Verification items for the finished model (mm, model axes). Face numbers are marked on the shaded views. A direction names the side the tool comes from. Round coordinates to 2 decimals unless told otherwise and drop trailing zeros. Write each loop counter-clockwise with the first axis right and the second up, starting at its lowest first coordinate (ties: lowest second). Pieces come first, ordered by that corner, then holes. Notation, with made-up numbers: M 83.25,34 L 127.25,34 A20 cw 127.25,48 Z; hole C 67.5,59 d7. An arc over 180 degrees is marked long. One line per question, with ' | ' between items. Start each with the question number.
Q1. Tool access check on the marked faces 4 and 5. Record the directions out of +Z, -Z, +X, -X, +Y, -Y that give a thin tool (end or side, any length) a straight path to the whole face; none if there is none.
Q2. Cross-section at C-C (x = -15). Record the boundary of the cut face in (y, z), then the cut area to 3 significant figures.
Q3. Cross-section at A-A (y = -2.75). Record the boundary of the cut face in (x, z).
Q4. Thickness scan on line 1 along X through (y, z) = (-9.5, -56.5); line 2 along Z through (x, y) = (17, -9.5); line 3 along X through (y, z) = (-13.25, -12.5). Record the ranges inside material, lowest first. Write a range as from..to.
Q5. Release check for a two-part mould opening along X. For the marked faces 1, 2 and 3 record: released by +X, released by -X, zero draft, split by the parting line, or undercut.
Q6. Gauge pin test, flat ends, axial feed: pin 1 (4 mm diameter, centred on x = 1.5, z = -57.5, fed in from -Y); pin 2 (2 mm diameter, centred on x = -6, y = -14.5, fed in from -Z). Record the tip position at first contact, or that the pin passes through.
Q7. Cross-section at D-D (z = -23.5). Record the boundary of the cut face in (x, y).
from build123d import *
from OCP.BRepFilletAPI import BRepFilletAPI_MakeChamfer

# Parameters (mm, degrees)
SKETCH1_W           = 35.4
SKETCH1_H           = 99.4
SKETCH1_W_2         = 33
SKETCH1_H_2         = 97
BOSS_EXTRUDE1_DEPTH = 2.4
SKETCH2_W           = 39.4
SKETCH2_H           = 103.4
SKETCH2_W_2         = 35.4
SKETCH2_H_2         = 99.4
BOSS_EXTRUDE3_DEPTH = 15.4
SKETCH3_W           = 39.4
SKETCH3_H           = 103.4
BOSS_EXTRUDE4_DEPTH = 2
BOSS_EXTRUDE5_DEPTH = 21.4
SKETCH5_R           = 5
CUT_EXTRUDE1_DEPTH  = 2.4
SKETCH6_W           = 4
SKETCH6_H           = 105.4
BOSS_EXTRUDE6_DEPTH = 1.6
CHAMFER1_SIZE       = 0.4
CHAMFER1_SIZE_2     = 2


with BuildPart() as part:
    # Sketch1 → Boss-Extrude1 (new body)
    with BuildSketch(Plane(origin=(0, 0, 0), x_dir=(1, 0, 0), z_dir=(0, 1, 0))):
        with Locations((0, 49.5)):
            Rectangle(SKETCH1_W, SKETCH1_H)
        with Locations((0, 49.5)):
            Rectangle(SKETCH1_W_2, SKETCH1_H_2, mode=Mode.SUBTRACT)
    extrude(amount=BOSS_EXTRUDE1_DEPTH)

    # Sketch2 → Boss-Extrude3 (add)
    with BuildSketch(Plane(origin=(0, 2.4, 0), x_dir=(1, 0, 0), z_dir=(0, 1, 0))):
        with Locations((0, 49.5)):
            Rectangle(SKETCH2_W, SKETCH2_H)
        with Locations((0, 49.5)):
            Rectangle(SKETCH2_W_2, SKETCH2_H_2, mode=Mode.SUBTRACT)
    extrude(amount=-BOSS_EXTRUDE3_DEPTH)

    # Sketch3 → Boss-Extrude4 (add)
    with BuildSketch(Plane(origin=(0, 2.4, 0), x_dir=(1, 0, 0), z_dir=(0, 1, 0))):
        with Locations((0, 49.5)):
            Rectangle(SKETCH3_W, SKETCH3_H)
    extrude(amount=BOSS_EXTRUDE4_DEPTH)

    # Sketch4 → Boss-Extrude5 (add)
    with BuildSketch(Plane(origin=(0, 4.4, 0), x_dir=(1, 0, 0), z_dir=(0, 1, 0))):
        Polygon((21.7, 101.2), (21.7, -4.2), (-21.7, -4.2), (-21.7, 101.2), (-19.7, 101.2), (-19.7, -2.2), (19.7, -2.2), (19.7, 101.2), align=None)
    extrude(amount=-BOSS_EXTRUDE5_DEPTH)

    # Sketch5 → Cut-Extrude1 (cut)
    with BuildSketch(Plane.XZ.offset(13)):
        with Locations((-15.2, -23.2)):
            Circle(SKETCH5_R)
        with Locations((15.2, -23.2)):
            Circle(SKETCH5_R)
        with Locations((15.2, -83.2)):
            Circle(SKETCH5_R)
        with Locations((-15.2, -83.2)):
            Circle(SKETCH5_R)
    extrude(amount=CUT_EXTRUDE1_DEPTH, mode=Mode.SUBTRACT)

    # Sketch6 → Boss-Extrude6 (add)
    with BuildSketch(Plane.XZ.offset(17)):
        with Locations((-19.7, -48.5)):
            Rectangle(SKETCH6_W, SKETCH6_H)
        with Locations((19.7, -48.5)):
            Rectangle(SKETCH6_W, SKETCH6_H)
    extrude(amount=-BOSS_EXTRUDE6_DEPTH)

    # Chamfer1
    chamfer1_edges_1 = [part.edges().sort_by_distance(p)[0] for p in [
        (17.7, -15.4, -49.5),
    ]]
    chamfer1_side_1 = [part.faces().sort_by_distance(p)[0] for p in [
        (17.7, -15.408, -49.5),
    ]]
    chamfer1_edges_2 = [part.edges().sort_by_distance(p)[0] for p in [
        (-17.7, -15.4, -49.5),
    ]]
    chamfer1_side_2 = [part.faces().sort_by_distance(p)[0] for p in [
        (-17.708, -15.4, -49.5),
    ]]
    chamfer1 = BRepFilletAPI_MakeChamfer(part.part.solid().wrapped)
    for e in chamfer1_edges_1:
        chamfer1.Add(CHAMFER1_SIZE - 0.0001, CHAMFER1_SIZE_2 - 0.0001, e.wrapped, chamfer1_side_1[0].wrapped)
    for e in chamfer1_edges_2:
        chamfer1.Add(CHAMFER1_SIZE_2 - 0.0001, CHAMFER1_SIZE - 0.0001, e.wrapped, chamfer1_side_2[0].wrapped)
    add(Compound.cast(chamfer1.Shape()), mode=Mode.REPLACE)  # a hair under: the kernel refuses the full size


solid = part.part
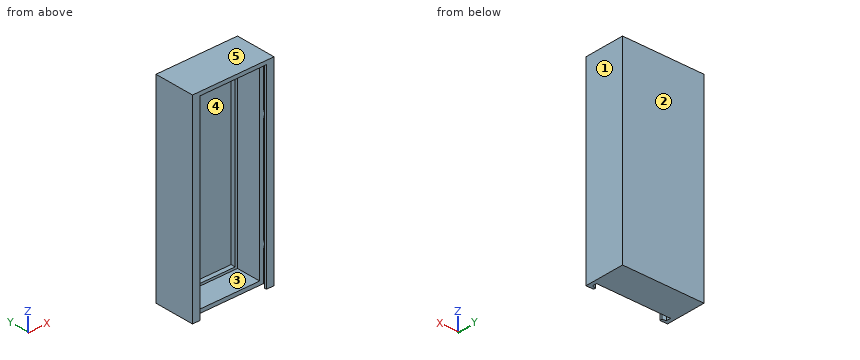
Determined:
1) face 4: -Y | face 5: +Z, +X, -X, +Y, -Y
2) outline: M -17,2.2 L -13,2.2 L -13,0.2 L 0,0.2 L 0,-1 L 2.4,-1 L 2.4,-98 L 0,-98 L 0,-99.2 L -13,-99.2 L -13,-101.2 L 4.4,-101.2 L 4.4,4.2 L -17,4.2 Z | area: 317 mm²
3) outline: M -21.7,-101.2 L 21.7,-101.2 L 21.7,4.2 L -21.7,4.2 Z; hole M -17.7,-99.2 L 17.7,-99.2 L 17.7,0.2 L -17.7,0.2 Z
4) line 1: x = -21.7..-17.7, 17.7..21.7 | line 2: z = -101.2..-99.2, 0.2..4.2 | line 3: x = -21.7..-19.7, 19.7..21.7
5) face 1: released by +X | face 2: zero draft | face 3: undercut
6) pin 1: stops at y = 2.4 | pin 2: stops at z = 2.2
7) outline: M -21.7,-17 L -17.7,-17 L -17.7,-15.8 L -19.7,-15.4 L -20.19,-15.4 L -20.19,-13 L -17.7,-13 L -17.7,0 L -16.5,0 L -16.5,2.4 L 16.5,2.4 L 16.5,0 L 17.7,0 L 17.7,-13 L 20.19,-13 L 20.19,-15.4 L 19.7,-15.4 L 17.7,-15.8 L 17.7,-17 L 21.7,-17 L 21.7,4.4 L -21.7,4.4 Z
